from build123d import *
from build123d.topology import SkipClean

# Parameters (mm, degrees)
SKETCH_1_W          = 62
SKETCH_1_H          = 45.22
EXTRUDE_1_DEPTH     = 4
SKETCH_7_W          = 62
SKETCH_7_H          = 4
EXTRUDE_4_DEPTH     = 4
SKETCH_2_R          = 1
CUT_EXTRUDE_1_DEPTH = 4
CUT_EXTRUDE_2_DEPTH = 1.2
FILLET_2_R          = 5
FILLET_4_R          = 5
FILLET_6_R          = 1
FILLET_7_R          = 1
FILLET_8_R          = 1
FILLET_9_R          = 1
SKETCH_3_R          = 2
CUT_EXTRUDE_6_DEPTH = 1.5
FILLET_10_R         = 5
FILLET_11_R         = 5
EXTRUDE_START       = 1
EXTRUDE_5_DEPTH     = 1


with BuildPart() as part:
    # Sketch 1 → Extrude 1 (new body)
    with BuildSketch(Plane.XY):
        with Locations((25.182910647, 19.462647059)):
            Rectangle(SKETCH_1_W, SKETCH_1_H)
    extrude(amount=EXTRUDE_1_DEPTH)

    # Sketch 7 → Extrude 4 (add)
    with BuildSketch(Plane(origin=(0, 42.072647059, 0), x_dir=(1, 0, 0), z_dir=(0, 1, 0))):
        with Locations((25.182910647, -2)):
            Rectangle(SKETCH_7_W, SKETCH_7_H)
    extrude(amount=EXTRUDE_4_DEPTH)

    # Sketch 2 → Cut-Extrude 1 (cut)
    with BuildSketch(Plane.XY.offset(4)):
        with BuildLine():
            ThreePointArc((18.542910647, 31.962647059), (2.852494887, 41.91252143), (0.542910647, 23.477365685))
            Line((0.542910647, 23.477365685), (0.542910647, 24.852647059))
            Line((0.542910647, 24.852647059), (14.542910647, 24.852647059))
            Line((14.542910647, 24.852647059), (14.542910647, 23.477365685))
            ThreePointArc((14.542910647, 23.477365685), (17.492785018, 27.272231299), (18.542910647, 31.962647059))
        make_face()
        with BuildLine():
            Line((0.542910647, 24.852647059), (0.542910647, 23.477365685))
            ThreePointArc((0.542910647, 23.477365685), (7.542910647, 20.962647059), (14.542910647, 23.477365685))
            Line((14.542910647, 23.477365685), (14.542910647, 24.852647059))
            Line((14.542910647, 24.852647059), (0.542910647, 24.852647059))
        make_face()
        with BuildLine():
            ThreePointArc((35.822910647, 23.477365685), (42.822910647, 20.962647059), (49.822910647, 23.477365685))
            Line((49.822910647, 23.477365685), (49.822910647, 24.852647059))
            Line((49.822910647, 24.852647059), (35.822910647, 24.852647059))
            Line((35.822910647, 24.852647059), (35.822910647, 23.477365685))
        make_face()
        with BuildLine():
            Line((49.822910647, 24.852647059), (49.822910647, 23.477365685))
            ThreePointArc((49.822910647, 23.477365685), (52.772785018, 27.272231299), (53.822910647, 31.962647059))
            ThreePointArc((53.822910647, 31.962647059), (38.132494887, 41.91252143), (35.822910647, 23.477365685))
            Line((35.822910647, 23.477365685), (35.822910647, 24.852647059))
            Line((35.822910647, 24.852647059), (49.822910647, 24.852647059))
        make_face()
        with Locations((-2.817089353, 23.662647059)):
            Circle(SKETCH_2_R)
        with Locations((17.902910647, 23.662647059)):
            Circle(SKETCH_2_R)
        with Locations((-2.817089353, 2.962647059)):
            Circle(SKETCH_2_R)
        with Locations((17.902910647, 2.962647059)):
            Circle(SKETCH_2_R)
        with Locations((32.462910647, 23.662647059)):
            Circle(SKETCH_2_R)
        with Locations((53.182910647, 23.662647059)):
            Circle(SKETCH_2_R)
        with Locations((53.182910647, 2.962647059)):
            Circle(SKETCH_2_R)
        with Locations((32.462910647, 2.962647059)):
            Circle(SKETCH_2_R)
    extrude(amount=-CUT_EXTRUDE_1_DEPTH, mode=Mode.SUBTRACT)

    # Sketch 2_3 → Cut-Extrude 2 (cut)
    with BuildSketch(Plane.XY.offset(4)):
        with BuildLine():
            Line((0.542910647, 23.477365685), (0.542910647, -3.147352941))
            Line((0.542910647, -3.147352941), (14.542910647, -3.147352941))
            Line((14.542910647, -3.147352941), (14.542910647, 23.477365685))
            ThreePointArc((14.542910647, 23.477365685), (7.542910647, 20.962647059), (0.542910647, 23.477365685))
        make_face()
        with BuildLine():
            Line((35.822910647, 23.477365685), (35.822910647, -3.147352941))
            Line((35.822910647, -3.147352941), (49.822910647, -3.147352941))
            Line((49.822910647, -3.147352941), (49.822910647, 23.477365685))
            ThreePointArc((49.822910647, 23.477365685), (42.822910647, 20.962647059), (35.822910647, 23.477365685))
        make_face()
    extrude(amount=-CUT_EXTRUDE_2_DEPTH, mode=Mode.SUBTRACT)

    # Fillet 2
    fillet_2_edges = [part.edges().sort_by_distance(p)[0] for p in [
        (-5.817089353, -3.147352941, 2),
    ]]
    fillet(fillet_2_edges, radius=FILLET_2_R)

    # Fillet 4
    fillet_4_edges = [part.edges().sort_by_distance(p)[0] for p in [
        (56.182910647, -3.147352941, 2),
    ]]
    fillet(fillet_4_edges, radius=FILLET_4_R)

    # Fillet 6
    fillet_6_edges = [part.edges().sort_by_distance(p)[0] for p in [
        (14.542910647, 10.165006372, 4),
    ]]
    fillet(fillet_6_edges, radius=FILLET_6_R)

    # Fillet 7
    fillet_7_edges = [part.edges().sort_by_distance(p)[0] for p in [
        (0.542910647, 10.165006372, 4),
    ]]
    fillet(fillet_7_edges, radius=FILLET_7_R)

    # Fillet 8
    fillet_8_edges = [part.edges().sort_by_distance(p)[0] for p in [
        (35.822910647, 10.165006372, 4),
    ]]
    fillet(fillet_8_edges, radius=FILLET_8_R)

    # Fillet 9
    fillet_9_edges = [part.edges().sort_by_distance(p)[0] for p in [
        (49.822910647, 10.165006372, 4),
    ]]
    fillet(fillet_9_edges, radius=FILLET_9_R)

    # Sketch 3 → Cut-Extrude 6 (cut)
    with BuildSketch(Plane(origin=(0, 0, 0), x_dir=(-1, 0, 0), z_dir=(0, 0, -1))):
        with Locations((-53.182910647, 2.962647059)):
            Circle(SKETCH_3_R)
        with Locations((-32.462910647, 2.962647059)):
            Circle(SKETCH_3_R)
        with Locations((-17.902910647, 2.962647059)):
            Circle(SKETCH_3_R)
        with Locations((2.817089353, 2.962647059)):
            Circle(SKETCH_3_R)
        with Locations((-53.182910647, 23.662647059)):
            Circle(SKETCH_3_R)
        with Locations((-32.462910647, 23.662647059)):
            Circle(SKETCH_3_R)
        with Locations((-17.902910647, 23.662647059)):
            Circle(SKETCH_3_R)
        with Locations((2.817089353, 23.662647059)):
            Circle(SKETCH_3_R)
    extrude(amount=-CUT_EXTRUDE_6_DEPTH, mode=Mode.SUBTRACT)

    # Fillet 10
    fillet_10_edges = [part.edges().sort_by_distance(p)[0] for p in [
        (56.182910647, 46.072647059, 2),
    ]]
    fillet(fillet_10_edges, radius=FILLET_10_R)

    # Fillet 11
    fillet_11_edges = [part.edges().sort_by_distance(p)[0] for p in [
        (-5.817089353, 46.072647059, 2),
    ]]
    fillet(fillet_11_edges, radius=FILLET_11_R)

    # Sketch 8 → Extrude 5 (add)
    with SkipClean():  # the faces are left unmerged after this step: merging them gives an invalid solid
        with BuildSketch(Plane.XY.offset(4).offset(EXTRUDE_START)):
            with BuildLine():
                Line((53.112123445, 28.072647059), (56.182910647, 28.072647059))
                Line((56.182910647, 28.072647059), (56.182910647, 41.072647059))
                ThreePointArc((56.182910647, 41.072647059), (54.718444553, 44.608180965), (51.182910647, 46.072647059))
                Line((51.182910647, 46.072647059), (-0.817089353, 46.072647059))
                ThreePointArc((-0.817089353, 46.072647059), (-4.352623259, 44.608180965), (-5.817089353, 41.072647059))
                Line((-5.817089353, 41.072647059), (-5.817089353, 28.072647059))
                Line((-5.817089353, 28.072647059), (-2.746302151, 28.072647059))
                ThreePointArc((-2.746302151, 28.072647059), (7.542910647, 42.962647059), (17.832123445, 28.072647059))
                Line((17.832123445, 28.072647059), (32.533697849, 28.072647059))
                ThreePointArc((32.533697849, 28.072647059), (42.822910647, 42.962647059), (53.112123445, 28.072647059))
            make_face()
        extrude(amount=-EXTRUDE_5_DEPTH)


solid = part.part
Check sheet for the modelled part. Datum: model origin and axes. Units: mm. A direction names the side the tool comes from. Coordinates: 2 decimals unless noted, no trailing zeros. Loops run counter-clockwise (first coordinate to the right, second up) from the corner with the lowest first, then second, coordinate; pieces in that order, holes last. Notation, with made-up numbers: (56, 13.25) -> (86, 13.25) arc R34 ccw to (86, 45.25) -> close; hole circle Ø8 at (14.25, -32). An arc over 180 degrees is marked (long way). Answer in a Markdown table with one row per item.
1. Sectioned sample at C-C, the plane x = 22.5. Record the boundary of the cut face in (y, z), then the cut area to 3 significant figures.
Check values:
| item | result |
|---|---|
| outline | (-3.15, 0) -> (46.07, 0) -> (46.07, 5) -> (28.07, 5) -> (28.07, 4) -> (-3.15, 4) -> close |
| area | 215 mm2 |
2. Material ranges on line 1 along X through (y, z) = (32, 2.1); line 2 along X through (y, z) = (13, 2.95); line 3 along Y through (x, z) = (31, 1.1), recorded low to high. Write a range as [from, to].
Check values:
| item | result |
|---|---|
| line 1 | x = [-5.82, -3.46], [18.54, 31.82], [53.82, 56.18] |
| line 2 | x = [-5.82, 0.54], [14.54, 35.82], [49.82, 56.18] |
| line 3 | y = [-3.15, 1.6], [4.33, 22.3], [25.03, 46.07] |
3. Access from +Z, -Z, +X, -X, +Y, -Y to the whole of each face (thin tool, end or side, straight path). Record for faces 1 (the face through (43, 10, 2.8)), 2 (the face through (25, 21, 0)), 3 (the face through (-3, 12, 4)), 4 (the face through (54.137, 3.263, 2.768)), 5 (the face through (30.555, 3.563, 0.74)).
Check values:
| item | result |
|---|---|
| face 1 | +Z, -Y |
| face 2 | -Z, +X, -X, +Y, -Y |
| face 3 | +Z, +X, -X, -Y |
| face 4 | +Z, -Z |
| face 5 | -Z |
4. Sectioned sample at B-B, the plane y = 6. Record the boundary of the cut face in (x, z), then the cut area to 3 significant figures.
Check values:
| item | result |
|---|---|
| outline | (-5.82, 0) -> (56.18, 0) -> (56.18, 4) -> (50.82, 4) arc R1 ccw to (49.82, 3) -> (49.82, 2.8) -> (35.82, 2.8) -> (35.82, 3) arc R1 ccw to (34.82, 4) -> (15.54, 4) arc R1 ccw to (14.54, 3) -> (14.54, 2.8) -> (0.54, 2.8) -> (0.54, 3) arc R1 ccw to (-0.46, 4) -> (-5.82, 4) -> close |
| area | 214 mm2 |
5. Sectioned sample at A-A, the plane x = 37. Record the boundary of the cut face in (y, z), then the cut area to 3 significant figures.
Check values:
| item | result |
|---|---|
| outline | (-3.15, 0) -> (22.63, 0) -> (22.63, 2.8) -> (-3.15, 2.8) -> close; (41.3, 0) -> (46.07, 0) -> (46.07, 5) -> (41.3, 5) -> close |
| area | 96.1 mm2 |
6. Go/stop test with flat-tipped pins: pin 1 (0.8 mm diameter, centred on x = -3.5, z = 4.5, fed in from -Y); pin 2 (3.5 mm diameter, centred on x = 17.9, y = 2.96, fed in from -Z); pin 3 (4.5 mm diameter, centred on x = -2.82, y = 23.66, fed in from +Z). Record where each tip stops, or that it passes through.
Check values:
| item | result |
|---|---|
| pin 1 | stops at y = 28.07 |
| pin 2 | stops at z = 1.5 |
| pin 3 | stops at z = 4 |
7. Release check for a two-part mould opening along X. For faces 6 (the face through (-4.391, -1.644, 2.028)), 7 (the face through (55.18, 3.05, 0.74)), 8 (the face through (25, 39, 5)) record: released by +X, released by -X, zero draft, split by the parting line, or undercut.
Check values:
| item | result |
|---|---|
| face 6 | released by -X |
| face 7 | undercut |
| face 8 | zero draft |
8. Sectioned sample at D-D, the plane y = 27. Record the boundary of the cut face in (x, z).
Check values:
| item | result |
|---|---|
| outline | (-5.82, 0) -> (-2.27, 0) -> (-2.27, 4) -> (-5.82, 4) -> close; (17.36, 0) -> (33.01, 0) -> (33.01, 4) -> (17.36, 4) -> close; (52.64, 0) -> (56.18, 0) -> (56.18, 4) -> (52.64, 4) -> close |
